Build history of the part. All positions in model axes, mm. Give positions to 0.01 mm unless a question says otherwise; leave off trailing zeros. Order: outer loops, then holes, each group sorted by start corner. A loop starts at its lowest first (then second) coordinate and runs counter-clockwise, first axis right, second up. Notation, with made-up numbers: (82, -7) - (141, -7) arc R14 cw to (141, 11) - close; hole circle Ø4 at (14.25, 79.5). An arc over 180 degrees is marked (long way). Answer in a Markdown table with one row per item.
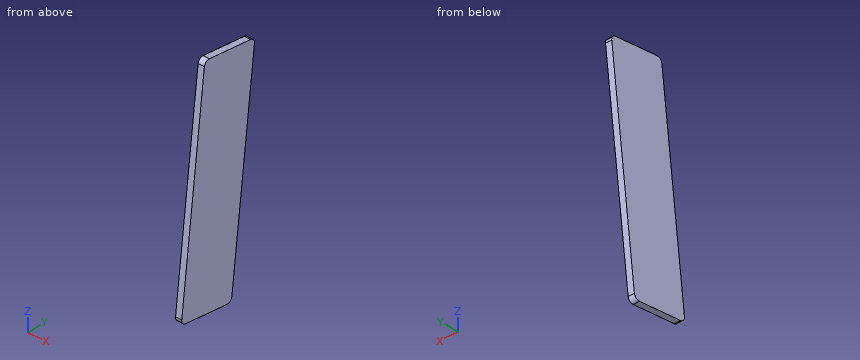
```python
from build123d import *

# Parameters (mm, degrees)
BOSS_EXTRUDE1_DEPTH = 2.5


with BuildPart() as part:
    # Sketch1 → Boss-Extrude1 (new body)
    with BuildSketch(Plane.ZY.offset(230.5)):
        with BuildLine():
            Line((-346.715127801, 353.841707564), (-344.651242875, 335.960421843))
            ThreePointArc((-344.651242875, 335.960421843), (-343.907165724, 334.622701789), (-342.435112803, 334.202932866))
            Line((-342.435112803, 334.202932866), (-257.002303251, 344.063716401))
            ThreePointArc((-257.002303251, 344.063716401), (-255.664583196, 344.807793551), (-255.244814273, 346.279846472))
            Line((-255.244814273, 346.279846472), (-257.308699199, 364.161132193))
            ThreePointArc((-257.308699199, 364.161132193), (-258.05277635, 365.498852247), (-259.524829271, 365.91862117))
            Line((-259.524829271, 365.91862117), (-344.957638824, 356.057837635))
            ThreePointArc((-344.957638824, 356.057837635), (-346.295358878, 355.313760485), (-346.715127801, 353.841707564))
        make_face()
    extrude(amount=BOSS_EXTRUDE1_DEPTH)


solid = part.part
```
1. Cut at A-A on x = -231.25. Write the cut outline in (y, z), and give its area (3 significant figures).
Check result:
| item | result |
|---|---|
| outline | (334.2, -342.44) arc R2 ccw to (335.96, -344.65) - (353.84, -346.72) arc R2 ccw to (356.06, -344.96) - (365.92, -259.52) arc R2 ccw to (364.16, -257.31) - (346.28, -255.24) arc R2 ccw to (344.06, -257) - close |
| area | 1,980 mm² |
2. Cut at B-B on z = -267.5. Write the cut outline in (x, y), and give its area (3 significant figures).
Check result:
| item | result |
|---|---|
| outline | (-233, 342.85) - (-230.5, 342.85) - (-230.5, 365) - (-233, 365) - close |
| area | 55.4 mm² |
3. Drop a flat-ended pin along its axis: P1, Ø1.5, axis at x = -232, y = 352.5, coming from the -Z side. Give the stop position or say it passes through.
Check result:
| item | result |
|---|---|
| P1 | stops at z = -346.65 |
4. Probe line 1 (Y direction, x = -231.85, z = -318); line 2 (Y direction, x = -232.8, z = -297); line 3 (Z direction, x = -231.8, y = 351). List the from-to ranges inside material, lowest first.
Check result:
| item | result |
|---|---|
| line 1 | y = 337.02 to 359.17 |
| line 2 | y = 339.45 to 361.59 |
| line 3 | z = -346.39 to -255.79 |
5. Cut at C-C on y = 361. Write the cut outline in (x, z), and give its area (3 significant figures).
Check result:
| item | result |
|---|---|
| outline | (-233, -302.14) - (-230.5, -302.14) - (-230.5, -256.94) - (-233, -256.94) - close |
| area | 113 mm² |
